from build123d import *

# Parameters (mm, degrees)
F4_W     = 3
F4_H     = 1
F6_R     = 1
F7_R     = 0.49999
F8_R     = 0.1
F9_DEPTH = 1


# Not quite as in the source:
# - a fillet or chamfer is up to 0.001 mm smaller than in the source, because OpenCascade refuses the exact size


with BuildPart() as f3:
    # F3: sweep along a path in F1
    with BuildLine(Plane.XZ) as f3_path:
        Line((0, 0), (0, -0.4))
    # F2 (on Top) → F3 (sweep)
    with BuildSketch(Plane.XY):
        Polygon((10.5, -7), (10.5, 1), (4.5, 1), (3.5, 1), (-10.5, 1), (-10.5, -7), (3.5, -7), (4.5, -7), align=None)
        Polygon((-7.9, -4.4), (-7.9, -1.6), (-4.5, -1.6), (4.5, -1.6), (7.9, -1.6), (7.9, -4.4), align=None, mode=Mode.SUBTRACT)
        with BuildLine():
            Line((3.5, 1), (4.5, 1))
            ThreePointArc((4.5, 1), (4, 1.5), (3.5, 1))
        make_face()
        with BuildLine():
            ThreePointArc((3.5, -7), (4, -7.5), (4.5, -7))
            Line((4.5, -7), (3.5, -7))
        make_face()
    sweep(path=f3_path.line)

    # F5: sweep along a path in F1
    with BuildLine(Plane.XZ) as f5_path:
        Line((0, 0), (0, 1))
    # F4 (on face) → F5 (sweep)
    with BuildSketch(Plane.XY):
        Polygon((4.5, 0), (9.5, 0), (9.5, -6), (10.5, -6), (10.5, 1), (4.5, 1), align=None)
        with Locations((3, 0.5)):
            Rectangle(F4_W, F4_H)
        Polygon((-9.5, -6), (-9.5, 0), (-9.5, 1), (-10.5, 1), (-10.5, -7), (-9.5, -7), align=None)
    sweep(path=f5_path.line)

    # F6
    f6_edges = [f3.edges().sort_by_distance(p)[0] for p in [
        (-7.9, -1.6, -0.2),
        (-7.9, -4.4, -0.2),
        (7.9, -1.6, -0.2),
        (7.9, -4.4, -0.2),
    ]]
    fillet(f6_edges, radius=F6_R)

    # F7 (radius 0.5 in the source; OpenCascade refuses exactly that, so slightly less here)
    f7_edges = [f3.edges().sort_by_distance(p)[0] for p in [
        (-10.5, -7, 0.3),
        (-10.5, 1, 0.3),
        (9.5, -6, 0.5),
        (10.5, -6, 0.5),
        (1.5, 0, 0.5),
        (10.5, -7, -0.2),
        (10.5, 1, 0.3),
        (1.5, 1, 0.5),
        (-9.5, 1, 0.5),
        (-9.5, -7, 0.5),
    ]]
    fillet(f7_edges, radius=F7_R)

    # F8 (on face) → F9 (cut, through all)
    with BuildSketch(Plane.XY.offset(1)):
        with Locations((9.5, 0)):
            Circle(F8_R)
    extrude(amount=-F9_DEPTH, mode=Mode.SUBTRACT)


solid = f3.part
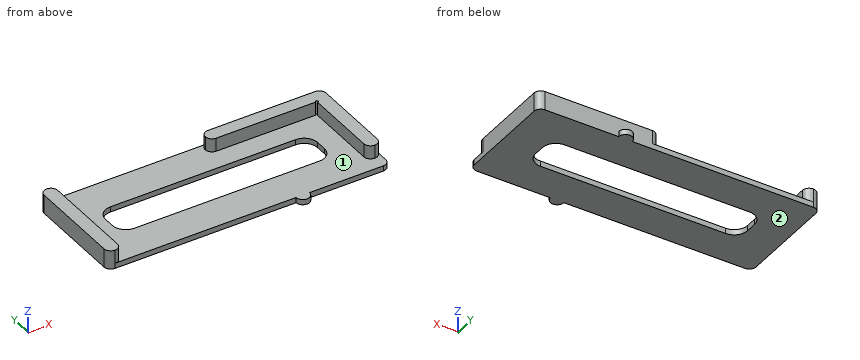
The model under review builds one solid part; all positions refer to its coordinate system, in mm. Face numbers are marked on the shaded views. Round coordinates to 2 decimals unless told otherwise and drop trailing zeros. Write each loop counter-clockwise with the first axis right and the second up, starting at its lowest first coordinate (ties: lowest second). Pieces come first, ordered by that corner, then holes. Notation, with made-up numbers: M 80,87.5 L 133,87.5 A22 cw 133,103.5 Z; hole C 65,63 d11. An arc over 180 degrees is marked long. Answer as CSV lines item,"result". Start each with the question number.
Q1. Consider section D-D, the plane x = 8.5. Give the boundary of the cut face in (y, z).
Q2. Consider section A-A, the plane x = 5. Give the boundary of the cut face in (y, z).
Q3. Clearance check with flat-ended pins moving along their axes: P1, Ø0.7, axis at x = -3, z = 0, coming from the +Y side; P2, Ø4, axis at x = -3.5, y = -3, coming from the +Z side. State where each tip first meets the part, or that it passes through.
Q4. Wall thickness on line 1 along X through (y, z) = (-2.25, 0.3); line 2 along Y through (x, z) = (5.75, -0.2); line 3 along Z through (x, y) = (-4.75, -4.75): over which ranges is each line inside the solid? List them lowest first.
Q5. Consider section C-C, the plane y = -2.25. Give the boundary of the cut face in (x, z).
Q6. The part is to be moulded in two halves that separate along X. For the marked faces 1 and 2, say which applies: +X half, -X half, draft (parallel to the pull), parting line (faces both ways), or undercut.
Result set:
1,outline,"M -7,-0.4 L 1,-0.4 L 1,1 L 0,1 L 0,0 L -7,0 Z"
2,outline,"M -7,-0.4 L -4.4,-0.4 L -4.4,0 L -7,0 Z; M -1.6,-0.4 L 1,-0.4 L 1,1 L 0,1 L 0,0 L -1.6,0 Z"
3,P1,"stops at y = 1"
3,P2,"stops at z = 0"
4,line 1,"x = -10.5 to -9.5, 9.5 to 10.5"
4,line 2,"y = -7 to -4.4, -1.6 to 1"
4,line 3,"z = -0.4 to 0"
5,outline,"M -10.5,-0.4 L -7.84,-0.4 L -7.84,0 L -9.5,0 L -9.5,1 L -10.5,1 Z; M 7.84,-0.4 L 10.5,-0.4 L 10.5,1 L 9.5,1 L 9.5,0 L 7.84,0 Z"
6,face 1,"undercut"
6,face 2,"draft"
